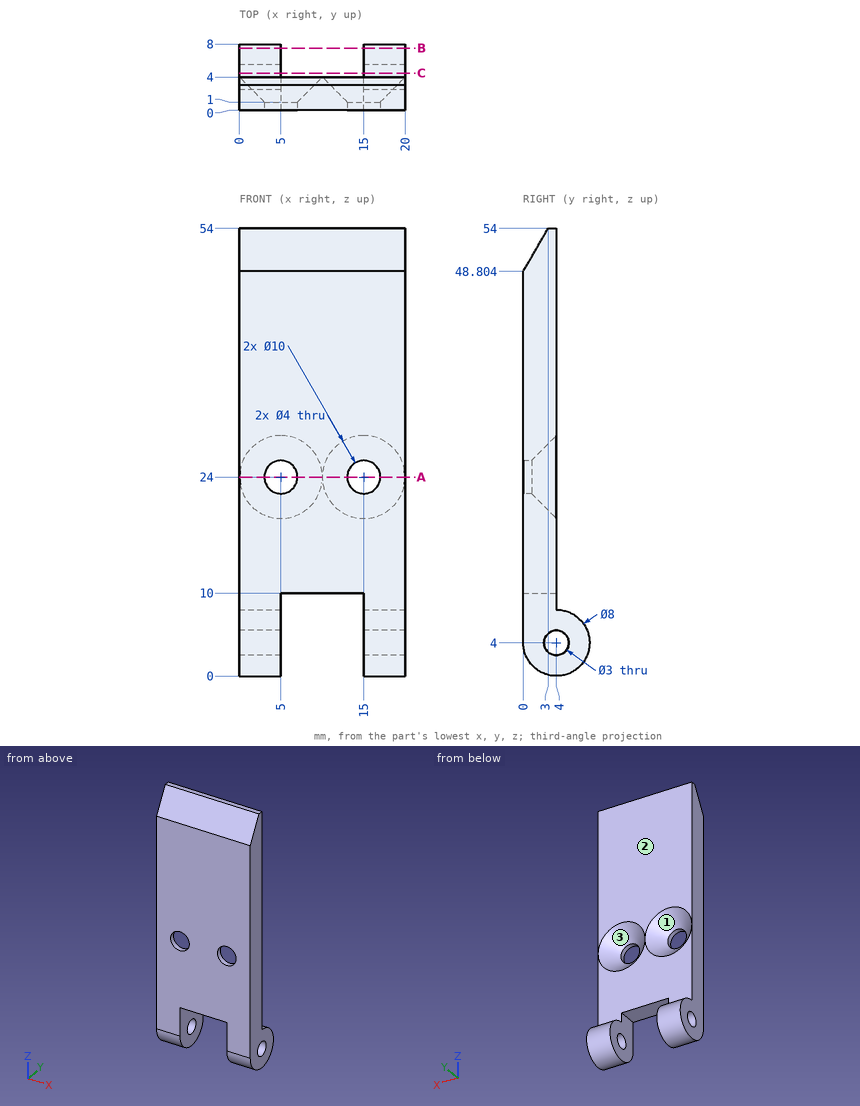
Input: dimensioned drawing with shaded views. Units: mm. Origin: part minimum x, y, z. Round coordinates to 2 decimals unless told otherwise and drop trailing zeros. Loops run counter-clockwise (first coordinate to the right, second up) from the corner with the lowest first, then second, coordinate; pieces in that order, holes last. Notation, with made-up numbers: (87.5, 76) -> (97.5, 76) arc R24 cw to (97.5, 93) -> close; hole circle Ø10 at (-6.75, 35). An arc over 180 degrees is marked (long way). One line per item, written item: value.
(1) Mould query, pull axis X, two halves, no side actions, for the marked faces 1, 2 and 3. Classes: pulls with the +X half, pulls with the -X half, needs draft (parallel to the pull), parting line crosses it, or undercut.
Geometry check:
face 1: undercut
face 2: needs draft
face 3: undercut
(2) Pin query (flat end, axial travel): pin 1 (10 mm diameter, centred on x = 10, z = 25, fed in from +Y); pin 2 (6.5 mm diameter, centred on x = 5, z = 24, fed in from +Y); pin 3 (3 mm diameter, centred on x = 2.5, y = 1, fed in from -Z). Return the tip coordinate at first contact, or that it passes through.
Geometry check:
pin 1: y = 4
pin 2: y = 2.25
pin 3: z = 0.29
(3) Material intervals for line 1 (X direction, y = 0.45, z = 24); line 2 (X direction, y = 2.5, z = 7); line 3 (Y direction, x = 17.25, z = 13), sorted ascending. Write a range as [from, to].
Geometry check:
line 1: [0, 3], [7, 13], [17, 20]
line 2: [0, 5], [15, 20]
line 3: [0, 4]
(4) Section C-C (y = 4.5). Return the cut outline in (x, z).
Geometry check:
outline: (0, 0.03) -> (5, 0.03) -> (5, 2.59) -> (0, 2.59) -> close; (0, 5.41) -> (5, 5.41) -> (5, 7.97) -> (0, 7.97) -> close; (15, 0.03) -> (20, 0.03) -> (20, 2.59) -> (15, 2.59) -> close; (15, 5.41) -> (20, 5.41) -> (20, 7.97) -> (15, 7.97) -> close
(5) Section B-B (y = 7.5). Return the cut outline in (x, z), plus the area to 3 significant figures.
Geometry check:
outline: (0, 2.06) -> (5, 2.06) -> (5, 5.94) -> (0, 5.94) -> close; (15, 2.06) -> (20, 2.06) -> (20, 5.94) -> (15, 5.94) -> close
area: 38.7 mm2
(6) Section A-A (z = 24). Give the number of separate pieces and of enclosed holes in the cut face, plus the area to 3 significant figures.
Geometry check:
separate pieces: 3
enclosed holes: 0
area: 30.0 mm2
